For this review, use the dimensioned drawing (mm, ordinates from the lowest corner) and the shaded views. Round coordinates to 2 decimals unless told otherwise and drop trailing zeros. Write each loop counter-clockwise with the first axis right and the second up, starting at its lowest first coordinate (ties: lowest second). Pieces come first, ordered by that corner, then holes. Notation, with made-up numbers: (-33.75, 71.5) -> (-21.75, 71.5) arc R27 cw to (-21.75, 102.5) -> close; hole circle Ø2 at (57, 70.5). An arc over 180 degrees is marked (long way). Write each question's results on one line, items separated by ' | '. Start each with the question number.
Item 1: Add section A-A (z = 8.5). State the section outline as (x, y) points.
Item 2: Add section B-B (z = 19). State the section outline as (x, y) points.
Item 3: Clearance check with flat-ended pins moving along their axes: pin 1 (5 mm diameter, centred on x = 9.5, z = 25, fed in from -Y); pin 2 (1 mm diameter, centred on y = 9.5, z = 35.5, fed in from -X); pin 3 (1 mm diameter, centred on x = 6.5, y = 7, fed in from -Z). State where each tip first meets the part, or that it passes through.
Item 4: To check wall thickness, follow line 1 along Y through (x, z) = (5.25, 30); line 2 along X through (y, z) = (1.5, 17); line 3 along X through (y, z) = (5, 37.5). State the ranges of each line that lie inside material, in increasing order.
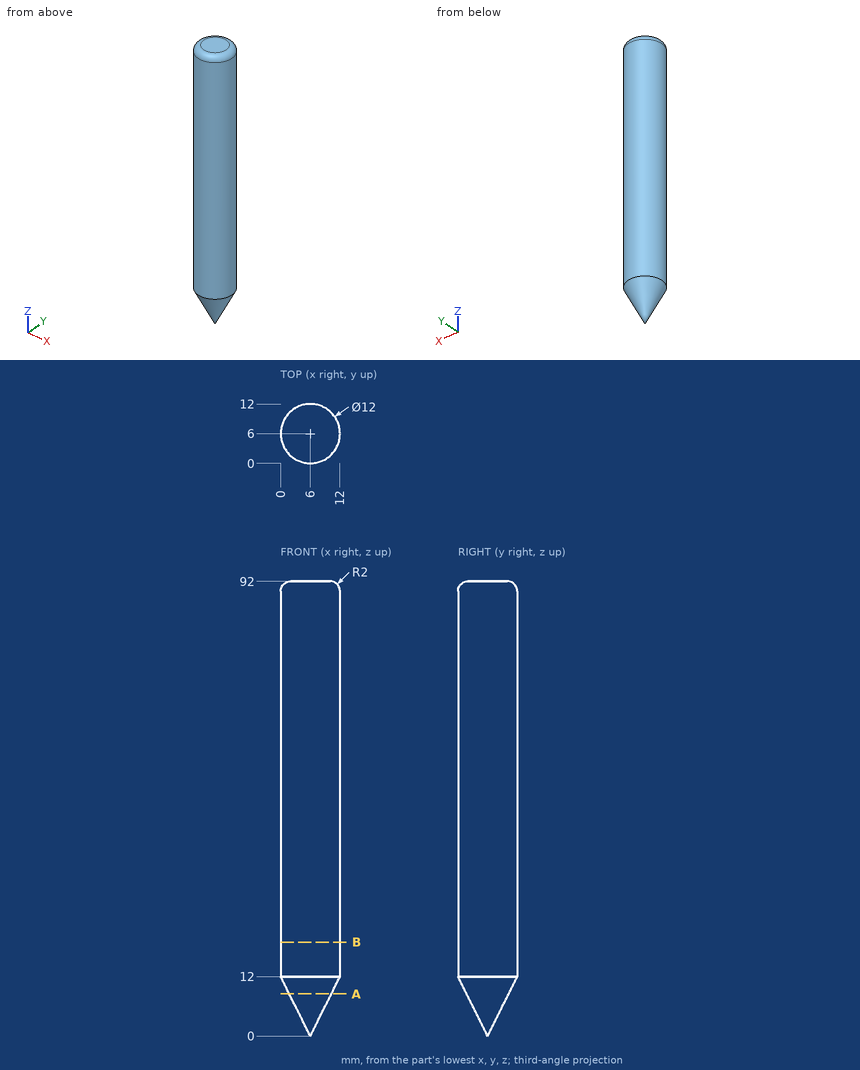
Responses:
1) outline: circle Ø8.5 at (6, 6)
2) outline: circle Ø12 at (6, 6)
3) pin 1: stops at y = 0.08 | pin 2: stops at x = 0.8 | pin 3: stops at z = 1.24
4) line 1: y = 0.05 to 11.95 | line 2: x = 2.03 to 9.97 | line 3: x = 0.08 to 11.92
